Could you check a few things on this model? Use its own coordinates, in mm. A direction names the side the tool comes from. Give positions to 0.01 mm unless a question says otherwise; leave off trailing zeros. Order: outer loops, then holes, each group sorted by start corner. A loop starts at its lowest first (then second) coordinate and runs counter-clockwise, first axis right, second up.
(1) Imagine slicing it at A-A, the plane x = -4. Write out the boundary of the cut face in (y, z), then the cut area to 3 significant figures.
(2) If we mould it in two halves opening along Z, with no side actions, what happens to faces 3 (the flat face through (4.35, 8, 0)), 4 (the flat face through (-8, 0, 6.45)), 5 (the conical face through (-10.44, -3.47, 11.017))? For each: released by +Z, released by -Z, zero draft, split by the parting line, or undercut.
(3) On a 3-axis mill with a long thin cutter (end or side, diameter ignored), from which of +Z, -Z, +X, -X, +Y, -Y can I reach the whole of each face in a straight line? I mean faces 1 (the flat face through (-8, 0, -6.45)), 2 (the flat face through (-25.65, 0, 0)). Say none if no direction works.
(4) If I drill on probe 1 along Z at (x, y) = (-9.5, -2); probe 2 along X at (y, z) = (-6.25, 3.75); probe 3 along Y at (x, z) = (-18, 5.25), over which ranges is the centre line in solid material (lowest first)?
(5) Imagine slicing it at C-C, the plane x = -23. Write out the boundary of the cut face in (y, z), then the cut area to 3 significant figures.
(6) Will these pins go through, and if not, where does the flat tip stop? pin 1 (6 mm diameter, centred on x = -18.5, y = 8.5, fed in from -Z); pin 2 (6.5 mm diameter, centred on x = -11.5, z = -2, fed in from -Y); pin 3 (10 mm diameter, centred on x = -16, z = 3, fed in from -Y).
(7) Imagine slicing it at B-B, the plane x = -11. Write out the boundary of the cut face in (y, z), then the cut area to 3 significant figures.
from build123d import *

# Parameters (mm, degrees)
SKETCH2_W          = 12.9
SKETCH2_H          = 12.9
CUT_EXTRUDE1_DEPTH = 25


with BuildPart() as part:
    # Sketch1 → Revolve1 (revolve)
    with BuildSketch(Plane.XY, mode=Mode.PRIVATE) as revolve1_sk:
        Polygon((-25.64984905, 0), (-25.64984905, -11.5), (4.35015095, -11.6), (4.35015095, 0), align=None)
    revolve(revolve1_sk.sketch.rotate(Axis((-25.64984905, 0, 0), (1, 0, 0)), 270), axis=Axis((-25.64984905, 0, 0), (1, 0, 0)))

    # Sketch2 → Cut-Extrude1 (cut)
    with BuildSketch(Plane(origin=(4.35015095, 0, 0), x_dir=(0, 0, -1), z_dir=(1, 0, 0))):
        Rectangle(SKETCH2_W, SKETCH2_H)
    extrude(amount=-CUT_EXTRUDE1_DEPTH, mode=Mode.SUBTRACT)


solid = part.part
Answer block:
1. outline: circle Ø23.14 at (0, 0); hole (-6.45, -6.45) - (6.45, -6.45) - (6.45, 6.45) - (-6.45, 6.45) - close
1. area: 254 mm2
2. face 3: zero draft
2. face 4: undercut
2. face 5: split by the parting line
3. face 1: +X
3. face 2: +Z, -Z, -X, +Y, -Y
4. probe 1: z = -11.38 to -6.45, 6.45 to 11.38
4. probe 2: x = -25.65 to -20.65
4. probe 3: y = -10.26 to -6.45, 6.45 to 10.26
5. outline: circle Ø23.02 at (0, 0)
5. area: 416 mm2
6. pin 1: stops at z = -10.13
6. pin 2: stops at y = -11.56
6. pin 3: stops at y = -11.55
7. outline: circle Ø23.1 at (0, 0); hole (-6.45, -6.45) - (6.45, -6.45) - (6.45, 6.45) - (-6.45, 6.45) - close
7. area: 253 mm2
